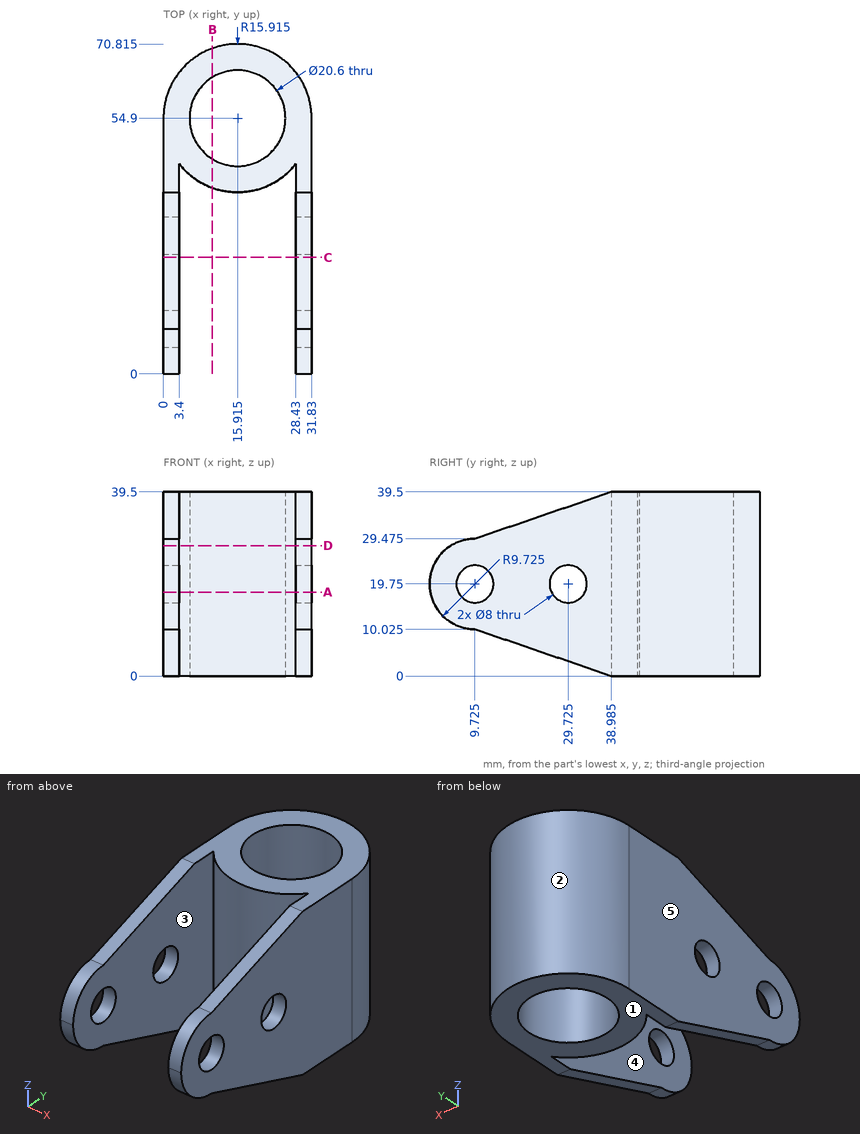
Answer from the drawing. Dimensions are ordinates in mm from the lowest x, y and z of the part. A direction names the side the tool comes from. Coordinates: 2 decimals unless noted, no trailing zeros. Order: outer loops, then holes, each group sorted by start corner. A loop starts at its lowest first (then second) coordinate and runs counter-clockwise, first axis right, second up. Notation, with made-up numbers: (-14.75, 44.5) - (0.25, 44.5) arc R25 cw to (0.25, 61.5) - close; hole circle Ø8 at (-8, 68). An arc over 180 degrees is marked (long way). Answer as a JSON object with one key per item and string values. Group by question number.
Item 1: Flat-ended cylindrical pins translate along their axes: P1, Ø5, axis at y = 9.725, z = 19.75, coming from the -X side; P2, Ø4, axis at x = 25, z = 33, coming from the -Y side; P3, Ø2, axis at y = 63, z = 20, coming from the -X side; P4, Ø4, axis at x = 22.5, z = 12.5, coming from the -Y side. Find the tip coordinate at first contact, or state that the pin passes through.
Item 2: Section A-A (z = 18) is taken. Give the vertices of the cut face in (x, y) (3 decimals), plus the area to 3 significant figures.
Item 3: Section B-B (x = 10.5) is taken. Give the vertices of the cut face in (y, z).
Item 4: Section D-D (z = 28) is taken. Give the vertices of the cut face in (x, y) (3 decimals).
Item 5: The mould has two halves that part along X. Classify the marked faces 1, 2 and 3: +X half, -X half, draft (parallel to the pull), parting line (faces both ways), or undercut.
Item 6: Section C-C (y = 25) is taken. Give the vertices of the cut face in (x, z).
Item 7: A tool of negligible diameter and unlimited length cuts with its end or side. For the marked faces 4 and 5, from which of +Z, -Z, +X, -X, +Y, -Y can it reach the whole face along a straight path? Write none if from no direction.
Item 8: Consider probe 1 along Y at (x, z) = (1.35, 19.75) (3 decimals); probe 2 along X at (y, z) = (38, 13.5); probe 3 along Y at (x, z) = (2, 19). Determine where each line is inside the solid, lowest interval first. Write a range as from..to.
Results are:
{
 "1": {"P1": "passes through", "P2": "stops at y = 40.65", "P3": "stops at x = 1.67", "P4": "stops at y = 39.66"},
 "2": {"outline": "(0, 0.159) - (3.4, 0.159) - (3.4, 6.128) - (0, 6.128) - close; (0, 13.322) - (3.4, 13.322) - (3.4, 26.128) - (0, 26.128) - close; (0, 33.322) - (3.4, 33.322) - (3.4, 45.068) arc R15.915 ccw to (28.43, 45.068) - (28.43, 33.322) - (31.83, 33.322) - (31.83, 54.9) arc R15.915 ccw to (0, 54.9) - close; (28.43, 0.159) - (31.83, 0.159) - (31.83, 6.128) - (28.43, 6.128) - close; (28.43, 13.322) - (31.83, 13.322) - (31.83, 26.128) - (28.43, 26.128) - close; hole circle Ø20.6 at (15.915, 54.9)", "area": "691 mm^2"},
 "3": {"outline": "(39.93, 0) - (46.14, 0) - (46.14, 39.5) - (39.93, 39.5) - close; (63.66, 0) - (69.87, 0) - (69.87, 39.5) - (63.66, 39.5) - close"},
 "4": {"outline": "(0, 4.576) - (3.4, 4.576) - (3.4, 45.068) arc R15.915 ccw to (28.43, 45.068) - (28.43, 4.576) - (31.83, 4.576) - (31.83, 54.9) arc R15.915 ccw to (0, 54.9) - close; hole circle Ø20.6 at (15.915, 54.9)"},
 "5": {"face 1": "draft", "face 2": "parting line", "face 3": "undercut"},
 "6": {"outline": "(0, 4.79) - (3.4, 4.79) - (3.4, 34.71) - (0, 34.71) - close; (28.43, 4.79) - (31.83, 4.79) - (31.83, 34.71) - (28.43, 34.71) - close"},
 "7": {"face 4": "+Z, -Z, -Y", "face 5": "+Z, -Z, -X, +Y, -Y"},
 "8": {"probe 1": "y = 0..5.725, 13.725..25.725, 33.725..61.315", "probe 2": "x = 0..3.4, 28.43..31.83", "probe 3": "y = 0.03..5.8, 13.65..25.8, 33.65..62.62"}
}
